Verification items for the finished model (mm, model axes). A direction names the side the tool comes from. Give positions to 0.01 mm unless a question says otherwise; leave off trailing zeros. Write each loop counter-clockwise with the first axis right and the second up, starting at its lowest first coordinate (ties: lowest second). Pieces come first, ordered by that corner, then holes. Notation, with made-up numbers: (51.5, -11.75) -> (94.5, -11.75) arc R10 ccw to (94.5, 1.25) -> close; hole circle Ø10 at (-16.5, 49.5). An arc over 180 degrees is marked (long way). Use one line per item in the form item = value. Start each with the question number.
(1) Section check B-B, the plane z = -3. Record the cut outline in (x, y).
(2) Set-up check for faces 1 (the face through (0, 7.5, 1)), 2 (the face through (29, 0, 1)), 3 (the face through (-29, 0, 1)): record each of +Z, -Z, +X, -X, +Y, -Y from which the full face is reachable in a straight line by a thin tool's end or side.
(3) Section check C-C, the plane y = 0. State how many separate pieces and enclosed holes the cut face has, plus the area to 3 significant figures.
(4) Section check D-D, the plane y = -5.75. Record the cut outline in (x, z), plus the area to 3 significant figures.
(5) Scan lines: L1, parallel to Y at x = 35, z = -1.9; L2, parallel to Y at x = -21, z = 1.45; L3, parallel to Z at x = 37.5, y = 3.25. Record each from-to range of solid material in increasing order.
(6) Section check A-A, the plane x = -21. Record the cut outline in (y, z), plus the area to 3 significant figures.
(7) Depth check by flat-ended pin: pin 1 Ø5 at (x, y) = (-21, 0) entering from +Z; pin 2 Ø8 at (x, y) = (35, 0) entering from +Z; pin 3 Ø6 at (x, y) = (21, 0) entering from -Z; pin 4 Ø1.2 at (y, z) = (-2.5, 1) entering from +X. Enter the tip coordinate at first touch or a pass-through.
(8) Release check for a two-part mould opening along Y. For faces 4 (the face through (0, -7.5, 1)), 5 (the face through (-42.5, 0, -2)), 6 (the face through (-25.995, 0.22, -4.803)) record: pulls with the +Y half, pulls with the -Y half, needs draft (parallel to the pull), parting line crosses it, or undercut.
from build123d import *

# Parameters (mm, degrees)
SKETCH_R       = 2.65
SKETCH_R_2     = 3.1
PAD_DEPTH      = 2
PAD_DEPTH_BACK = 5
SKETCH001_W    = 85
SKETCH001_H    = 26
POCKET_DEPTH   = 5
FILLET_R       = 5
CHAMFER_SIZE   = 0.5


with BuildPart() as part:
    # Sketch → Pad (new body, two sides)
    with BuildSketch(Plane.XY) as pad_sk:
        with BuildLine():
            Line((-42.5, 13), (-0.5, 13))
            ThreePointArc((-0.5, 13), (0, 12.5), (0.5, 13))
            Line((0.5, 13), (42.5, 13))
            Line((42.5, 13), (42.5, -13))
            Line((42.5, -13), (-42.5, -13))
            Line((-42.5, -13), (-42.5, 13))
        make_face()
        with Locations((-21, 0)):
            Circle(SKETCH_R, mode=Mode.SUBTRACT)
        with Locations((-35, 0)):
            Circle(SKETCH_R_2, mode=Mode.SUBTRACT)
        with Locations((35, 0)):
            Circle(SKETCH_R_2, mode=Mode.SUBTRACT)
        with Locations((21, 0)):
            Circle(SKETCH_R, mode=Mode.SUBTRACT)
    extrude(amount=PAD_DEPTH)
    extrude(pad_sk.sketch, amount=-PAD_DEPTH_BACK)

    # Sketch001 → Pocket (cut)
    with BuildSketch(Plane.XY):
        Rectangle(SKETCH001_W, SKETCH001_H)
        with BuildLine():
            Line((-28.5, 7.5), (28.5, 7.5))
            ThreePointArc((29, 7), (28.853553, 7.353553), (28.5, 7.5))
            Line((29, 7), (29, -7))
            ThreePointArc((28.5, -7.5), (28.853553, -7.353553), (29, -7))
            Line((28.5, -7.5), (-28.5, -7.5))
            ThreePointArc((-29, -7), (-28.853553, -7.353553), (-28.5, -7.5))
            Line((-29, -7), (-29, 7))
            ThreePointArc((-28.5, 7.5), (-28.853553, 7.353553), (-29, 7))
        make_face(mode=Mode.SUBTRACT)
    extrude(amount=POCKET_DEPTH, mode=Mode.SUBTRACT)

    # Sketch002 → Groove (revolve, cut)
    with BuildSketch(Plane.XZ):
        Polygon((-21, 0.4), (-16, -4.6), (-16, -5), (-21, -5), align=None)
    revolve(axis=Axis((-21, 0, 0), (0, 0, 1)), mode=Mode.SUBTRACT)

    # Sketch003 → Groove001 (revolve, cut)
    with BuildSketch(Plane.XZ):
        Polygon((21, 0.4), (26, -4.6), (26, -5), (21, -5), align=None)
    revolve(axis=Axis((21, 0, 0), (0, 0, 1)), mode=Mode.SUBTRACT)

    # Fillet
    fillet_edges = [part.edges().sort_by_distance(p)[0] for p in [
        (42.5, 13, -2.5),
        (42.5, -13, -2.5),
        (-42.5, 13, -2.5),
        (-42.5, -13, -2.5),
    ]]
    fillet(fillet_edges, radius=FILLET_R)

    # Chamfer
    chamfer_edges = [part.edges().sort_by_distance(p)[0] for p in [
        (0, 7.5, 0),
    ]]
    chamfer(chamfer_edges, length=CHAMFER_SIZE)


solid = part.part
Completed:
q1.outline = (-42.5, -8) arc R5 ccw to (-37.5, -13) -> (37.5, -13) arc R5 ccw to (42.5, -8) -> (42.5, 8) arc R5 ccw to (37.5, 13) -> (0.5, 13) arc R0.5 cw to (-0.5, 13) -> (-37.5, 13) arc R5 ccw to (-42.5, 8) -> close; hole circle Ø6.2 at (-35, 0); hole circle Ø6.8 at (-21, 0); hole circle Ø6.8 at (21, 0); hole circle Ø6.2 at (35, 0)
q2.face_1 = +Z, +X, -X, +Y
q2.face_2 = +Z, +X, +Y, -Y
q2.face_3 = +Z, -X, +Y, -Y
q3.separate_pieces = 5
q3.enclosed_holes = 0
q3.area = 390 mm²
q4.outline = (-42.5, -5) -> (42.5, -5) -> (42.5, 0) -> (29.5, 0) -> (29, 0.5) -> (29, 2) -> (-29, 2) -> (-29, 0.5) -> (-29.5, 0) -> (-42.5, 0) -> close
q4.area = 541 mm²
q5.L1 = -13 to -3.1, 3.1 to 13
q5.L2 = -7.5 to -2.65, 2.65 to 7.5
q5.L3 = -5 to 0
q6.outline = (-13, -5) -> (-5, -5) -> (-5, -4.6) -> (-2.65, -2.25) -> (-2.65, 2) -> (-7.5, 2) -> (-7.5, 0.5) -> (-8, 0) -> (-13, 0) -> close; (2.65, -2.25) -> (5, -4.6) -> (5, -5) -> (13, -5) -> (13, 0) -> (8, 0) -> (7.5, 0.5) -> (7.5, 2) -> (2.65, 2) -> close
q6.area = 116 mm²
q7.pin_1 = through
q7.pin_2 = 0
q7.pin_3 = -2.6
q7.pin_4 = 29.1
q8.face_4 = pulls with the -Y half
q8.face_5 = needs draft
q8.face_6 = undercut
